```python
from build123d import *

# Parameters (mm, degrees)
SKETCH_1_R          = 29.4
SKETCH_1_R_2        = 2.25
EXTRUDE_1_DEPTH     = 13.9
SKETCH_2_OUTSIDE_W  = 77.662
SKETCH_2_OUTSIDE_H  = 77.662
SKETCH_2_OUTSIDE_R  = 11
CUT_EXTRUDE_1_DEPTH = 44.83982208
FILLET_1_R          = 10


with BuildPart() as part:
    # 草图1 → 凸台-拉伸1 (new body)
    with BuildSketch(Plane.XY):
        Circle(SKETCH_1_R)
        with Locations((-17.25, 0)):
            Circle(SKETCH_1_R_2, mode=Mode.SUBTRACT)
        with Locations((-8.625, 14.938938215)):
            Circle(SKETCH_1_R_2, mode=Mode.SUBTRACT)
        with Locations((8.625, 14.938938215)):
            Circle(SKETCH_1_R_2, mode=Mode.SUBTRACT)
        with Locations((17.25, 0)):
            Circle(SKETCH_1_R_2, mode=Mode.SUBTRACT)
        with Locations((8.625, -14.938938215)):
            Circle(SKETCH_1_R_2, mode=Mode.SUBTRACT)
        with Locations((-8.625, -14.938938215)):
            Circle(SKETCH_1_R_2, mode=Mode.SUBTRACT)
    extrude(amount=EXTRUDE_1_DEPTH)

    # 草图2 outside → 切除-拉伸1 (cut, through all)
    # profile 1 of 2: a face of its own
    with BuildSketch(Plane.XY.offset(13.9)):
        Rectangle(SKETCH_2_OUTSIDE_W, SKETCH_2_OUTSIDE_H)
        Polygon((12.990381057, 22.5), (-12.990381057, 22.5), (-25.980762114, 0), (-12.990381057, -22.5), (12.990381057, -22.5), (25.980762114, 0), align=None, mode=Mode.SUBTRACT)
    # profile 2 of 2: a face of its own
    with BuildSketch(Plane.XY.offset(13.9)):
        Circle(SKETCH_2_OUTSIDE_R)
    extrude(amount=-CUT_EXTRUDE_1_DEPTH, mode=Mode.SUBTRACT)

    # 圆角1
    fillet_1_edges = [part.edges().sort_by_distance(p)[0] for p in [
        (25.980762114, 0, 6.95),
        (12.990381057, -22.5, 6.95),
        (-12.990381057, -22.5, 6.95),
        (-25.980762114, 0, 6.95),
        (-12.990381057, 22.5, 6.95),
        (12.990381057, 22.5, 6.95),
    ]]
    fillet(fillet_1_edges, radius=FILLET_1_R)


solid = part.part
```
Input: part model. Units: mm. Frame: model coordinates. Round coordinates to 2 decimals unless told otherwise and drop trailing zeros. Write each loop counter-clockwise with the first axis right and the second up, starting at its lowest first coordinate (ties: lowest second). Pieces come first, ordered by that corner, then holes. Notation, with made-up numbers: (8, 54) -> (29, 54) arc R9 ccw to (29, 58) -> close; hole circle Ø6 at (-31.75, 13.5). An arc over 180 degrees is marked (long way). Answer as CSV lines item,"result".
1. Section A-A (x = 0). Return the cut outline in (y, z).
Geometry says:
outline,"(-22.5, 0) -> (-11, 0) -> (-11, 13.9) -> (-22.5, 13.9) -> close; (11, 0) -> (22.5, 0) -> (22.5, 13.9) -> (11, 13.9) -> close"
2. Ray query, L1, parallel to Y at x = 0, z = 8.75; L2, parallel to Y at x = -5, z = 12.75; L3, parallel to Y at x = -10, z = 12. Return the intervals inside material, ascending. Write a range as [from, to].
Geometry says:
L1,"y = [-22.5, -11], [11, 22.5]"
L2,"y = [-22.5, -9.8], [9.8, 22.5]"
L3,"y = [-22.1, -16.72], [-13.16, -4.58], [4.58, 13.16], [16.72, 22.1]"
3. Section B-B (y = 0). Return the cut outline in (x, z), plus the area to 3 significant figures.
Geometry says:
outline,"(-24.43, 0) -> (-19.5, 0) -> (-19.5, 13.9) -> (-24.43, 13.9) -> close; (-15, 0) -> (-11, 0) -> (-11, 13.9) -> (-15, 13.9) -> close; (11, 0) -> (15, 0) -> (15, 13.9) -> (11, 13.9) -> close; (19.5, 0) -> (24.43, 0) -> (24.43, 13.9) -> (19.5, 13.9) -> close"
area,"248 mm^2"
4. Mould query, pull axis Y, two halves, no side actions, for faces 1 (the cylindrical face through (-2.38, -10.74, 7.05)), 2 (the cylindrical face through (12.28, 21.123, 6.853)), 3 (the cylindrical face through (12.28, -21.123, 6.853)). Classes: +Y half, -Y half, draft (parallel to the pull), parting line (faces both ways), or undercut.
Geometry says:
face 1,"undercut"
face 2,"+Y half"
face 3,"-Y half"
5. Section D-D (z = 11.75). Return the cut outline in (x, y) (3 decimals).
Geometry says:
outline,"(-23.094, -5) -> (-15.877, -17.5) arc R10 ccw to (-7.217, -22.5) -> (7.217, -22.5) arc R10 ccw to (15.877, -17.5) -> (23.094, -5) arc R10 ccw to (23.094, 5) -> (15.877, 17.5) arc R10 ccw to (7.217, 22.5) -> (-7.217, 22.5) arc R10 ccw to (-15.877, 17.5) -> (-23.094, 5) arc R10 ccw to start; hole circle Ø4.5 at (-17.25, 0); hole circle Ø22 at (0, 0); hole circle Ø4.5 at (-8.625, -14.939); hole circle Ø4.5 at (-8.625, 14.939); hole circle Ø4.5 at (8.625, -14.939); hole circle Ø4.5 at (8.625, 14.939); hole circle Ø4.5 at (17.25, 0)"
6. Contact query for flat-ended pins moving along their axis: P1, Ø4, axis at x = -7.5, z = 2.5, coming from the -Y side; P2, Ø4, axis at y = -5, z = 11.5, coming from the -X side; P3, Ø4, axis at y = -6.5, z = 8.5, coming from the -X side. Output: stop coordinate, or through.
Geometry says:
P1,"stops at y = -22.5"
P2,"stops at x = -23.97"
P3,"stops at x = -23.36"
7. Section C-C (y = 8). Return the cut outline in (x, z).
Geometry says:
outline,"(-21.36, 0) -> (-7.55, 0) -> (-7.55, 13.9) -> (-21.36, 13.9) -> close; (7.55, 0) -> (21.36, 0) -> (21.36, 13.9) -> (7.55, 13.9) -> close"
